```python
from build123d import *

# Parameters (mm, degrees)
SKETCH1_R           = 1.5
BOSS_EXTRUDE1_DEPTH = 7.9
SKETCH3_W           = 2.5
SKETCH3_H           = 2.95
CUT_EXTRUDE1_DEPTH  = 1.778


with BuildPart() as part:
    # Sketch1 → Boss-Extrude1 (new body)
    with BuildSketch(Plane(origin=(0, 0, 0), x_dir=(1, 0, 0), z_dir=(0, 1, 0))):
        Circle(SKETCH1_R)
    extrude(amount=BOSS_EXTRUDE1_DEPTH)

    # Sketch3 → Revolve1 (revolve)
    with BuildSketch(Plane.XY):
        with Locations((1.25, 9.375)):
            Rectangle(SKETCH3_W, SKETCH3_H)
    revolve(axis=Axis((0, 7.9, 0), (0, 1, 0)))

    # Sketch4 → Cut-Extrude1 (cut)
    with BuildSketch(Plane(origin=(0, 10.85, 0), x_dir=(1, 0, 0), z_dir=(0, 1, 0))):
        Polygon((1.443375673, 0), (0.721687836, 1.25), (-0.721687836, 1.25), (-1.443375673, 0), (-0.721687836, -1.25), (0.721687836, -1.25), align=None)
    extrude(amount=-CUT_EXTRUDE1_DEPTH, mode=Mode.SUBTRACT)


solid = part.part
```
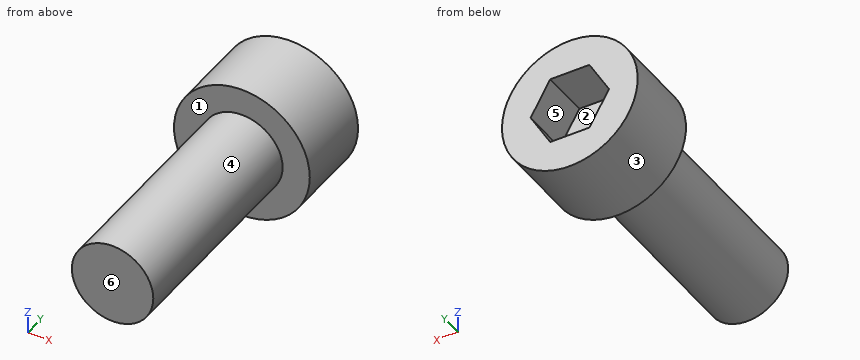
For this review, take the finished solid that the model builds, in its own axes (mm). Face numbers are marked on the shaded views. A direction names the side the tool comes from. Give positions to 0.01 mm unless a question says otherwise; leave off trailing zeros. Write each loop counter-clockwise with the first axis right and the second up, starting at its lowest first coordinate (ties: lowest second). Pieces come first, ordered by that corner, then holes. Notation, with made-up numbers: M -21,-19.75 L 11,-19.75 A10 cw 11,-2.75 Z; hole C 2,-29.75 d4. An arc over 180 degrees is marked long. One line per item, written item: value.
1) For line 1 (Y direction, x = 1.75, z = -0.05); line 2 (X direction, y = 10.25, z = -1.05); line 3 (Y direction, x = -0.95, z = -0.7), list the stretches that pass through material, from the lowest coordinate up. Write a range as from..to.
Results are:
line 1: y = 7.9..10.85
line 2: x = -2.27..-0.84, 0.84..2.27
line 3: y = 0..9.07
2) The part is to be moulded in two halves that separate along Z. For the marked faces 1, 2 and 3, say which applies: +Z half, -Z half, draft (parallel to the pull), parting line (faces both ways), or undercut.
Results are:
face 1: draft
face 2: undercut
face 3: parting line
3) Take a section at C-C, the plane z = 0.75. Write out the cut boundary in (x, y).
Results are:
outline: M -2.38,7.9 L -1.3,7.9 L -1.3,0 L 1.3,0 L 1.3,7.9 L 2.38,7.9 L 2.38,10.85 L 1.01,10.85 L 1.01,9.07 L -1.01,9.07 L -1.01,10.85 L -2.38,10.85 Z
4) For P1, Ø1, axis at x = -0.5, z = -2, coming from the -Y side; P2, Ø1, axis at x = -1, y = 9.5, coming from the -Z side; P3, Ø3, axis at x = 0.5, z = 0, coming from the +Y side; P4, Ø3, axis at x = 0, y = 2, coming from the +Z side, all flat-tipped, find the tip position at first contact; note any pin that passes through.
Results are:
P1: stops at y = 7.9
P2: stops at z = -2.45
P3: stops at y = 10.85
P4: stops at z = 1.5
5) For the marked faces 4, 5 and 6, list the 3-axis set-ups (+Z, -Z, +X, -X, +Y, -Y) from which the entire face can be reached by the end or side of a thin tool; tool diameter is ignored.
Results are:
face 4: -Y
face 5: +Y
face 6: +Z, -Z, +X, -X, -Y
6) Take a section at A-A, the plane y = 9.75. Write out the cut boundary in (x, z).
Results are:
outline: C 0,0 d5; hole M -1.44,0 L -0.72,-1.25 L 0.72,-1.25 L 1.44,0 L 0.72,1.25 L -0.72,1.25 Z
7) Take a section at D-D, the plane y = 4.25. Write out the cut boundary in (x, z).
Results are:
outline: C 0,0 d3
8) Take a section at B-B, the plane x = 0. Write out the cut boundary in (y, z).
Results are:
outline: M 0,-1.5 L 7.9,-1.5 L 7.9,-2.5 L 10.85,-2.5 L 10.85,-1.25 L 9.07,-1.25 L 9.07,1.25 L 10.85,1.25 L 10.85,2.5 L 7.9,2.5 L 7.9,1.5 L 0,1.5 Z
